The listing builds one solid part. Answer for the finished solid, in the listing's coordinates (mm). Face numbers are marked on the shaded views. A direction names the side the tool comes from. Round coordinates to 2 decimals unless told otherwise and drop trailing zeros. Write each loop counter-clockwise with the first axis right and the second up, starting at its lowest first coordinate (ties: lowest second). Pieces come first, ordered by that corner, then holes. Notation, with made-up numbers: (66.5, -8.5) - (92.5, -8.5) arc R20 ccw to (92.5, -1.5) - close; hole circle Ø1 at (5, -9). An arc over 180 degrees is marked (long way). Answer as CSV lines item,"result". Start each with the question number.
Item 1: A cutting plane is placed at D-D on z = 42. Determine the outline of the cut face in (x, y), and give its area (3 significant figures).
Item 2: Flat-ended cylindrical pins translate along their axes: pin 1 (3 mm diameter, centred on x = -52.75, y = -52.75, fed in from +Z) (3 decimals); pin 2 (2 mm diameter, centred on x = 10.5, y = 19, fed in from +Z); pin 3 (12 mm diameter, centred on x = -2, y = 4, fed in from +Z); pin 4 (5 mm diameter, centred on y = 22, z = 11.5, fed in from +X). Find the tip coordinate at first contact, or state that the pin passes through.
Item 3: A cutting plane is placed at A-A on z = 66.5. Determine the outline of the cut face in (x, y), and give its area (4 significant figures).
Item 4: A cutting plane is placed at B-B on x = 21.5. Determine the outline of the cut face in (y, z).
Item 5: A cutting plane is placed at C-C on y = 28. State how many separate pieces and enclosed holes the cut face has, and give its area (3 significant figures).
Item 6: Which of the six approach directions +Z, -Z, +X, -X, +Y, -Y give full straight-line access (tool end or side, diameter ignored) to the marked faces 1, 2 and 3?
Item 7: Straight lines are drawn through the part: line 1 along Y through (x, z) = (52.75, 1.15); line 2 along Z through (x, y) = (-13, 28.5); line 3 along X through (y, z) = (52, 1). For each, find the intervals that lie inside material, in ascending order. Write a range as [from, to].
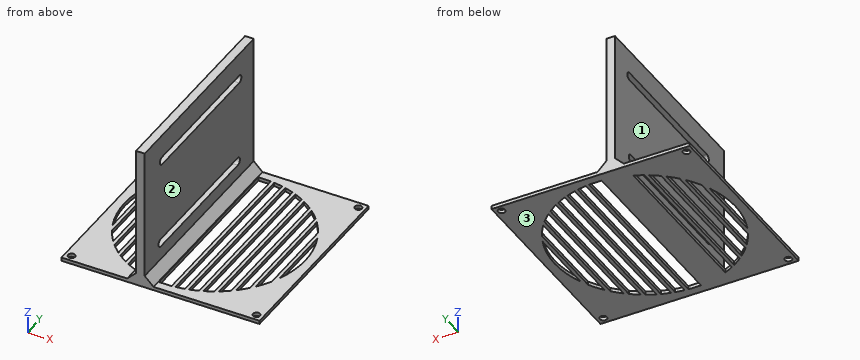
```python
from build123d import *

# Parameters (mm, degrees)
F0_W     = 113
F0_H     = 113
F0_R     = 2
F0_W_2   = 7.1751601063
F0_H_2   = 103.030346334
F1_DEPTH = 2
F2_W     = 5
F2_H     = 113
F3_DEPTH = 80
F5_DEPTH = 25
F6_SIZE  = 5


with BuildPart() as f1:
    # F0 (on Top) → F1 (new body)
    with BuildSketch(Plane.XY):
        Rectangle(F0_W, F0_H)
        with Locations((-52.75, -52.75)):
            Circle(F0_R, mode=Mode.SUBTRACT)
        with BuildLine():
            ThreePointArc((-47.5875800531, -19.6893937105), (-51.5, 0), (-47.5875800531, 19.6893937105))
            Line((-47.5875800531, 19.6893937105), (-47.5875800531, -19.6893937105))
        make_face(mode=Mode.SUBTRACT)
        with Locations((52.75, -52.75)):
            Circle(F0_R, mode=Mode.SUBTRACT)
        with BuildLine():
            Line((45.5875800531, 23.9587675998), (45.5875800531, -23.9587675998))
            ThreePointArc((45.5875800531, -23.9587675998), (43.2610879903, -27.9415150967), (40.5875800531, -31.7001316311))
            Line((40.5875800531, -31.7001316311), (40.5875800531, 31.7001316311))
            ThreePointArc((40.5875800531, 31.7001316311), (43.2610879903, 27.9415150967), (45.5875800531, 23.9587675998))
        make_face(mode=Mode.SUBTRACT)
        with BuildLine():
            Line((-45.5875800531, -23.9587675998), (-45.5875800531, 23.9587675998))
            ThreePointArc((-45.5875800531, 23.9587675998), (-43.2610879903, 27.9415150967), (-40.5875800531, 31.7001316311))
            Line((-40.5875800531, 31.7001316311), (-40.5875800531, -31.7001316311))
            ThreePointArc((-40.5875800531, -31.7001316311), (-43.2610879903, -27.9415150967), (-45.5875800531, -23.9587675998))
        make_face(mode=Mode.SUBTRACT)
        with BuildLine():
            Line((-38.5875800531, -34.106431441), (-38.5875800531, 34.106431441))
            ThreePointArc((-38.5875800531, 34.106431441), (-36.1717921774, 36.6585794962), (-33.5875800531, 39.0400367082))
            Line((-33.5875800531, 39.0400367082), (-33.5875800531, -39.0400367082))
            ThreePointArc((-33.5875800531, -39.0400367082), (-36.1717921774, -36.6585794962), (-38.5875800531, -34.106431441))
        make_face(mode=Mode.SUBTRACT)
        with BuildLine():
            Line((-31.5875800531, -40.6752355419), (-31.5875800531, 40.6752355419))
            ThreePointArc((-31.5875800531, 40.6752355419), (-29.1381205687, 42.4643371516), (-26.5875800531, 44.1061286775))
            Line((-26.5875800531, 44.1061286775), (-26.5875800531, -44.1061286775))
            ThreePointArc((-26.5875800531, -44.1061286775), (-29.1381205687, -42.4643371516), (-31.5875800531, -40.6752355419))
        make_face(mode=Mode.SUBTRACT)
        with BuildLine():
            Line((-24.5875800531, -45.2515293347), (-24.5875800531, 45.2515293347))
            ThreePointArc((-24.5875800531, 45.2515293347), (-22.1195608355, 46.5077953513), (-19.5875800531, 47.6295780756))
            Line((-19.5875800531, 47.6295780756), (-19.5875800531, -47.6295780756))
            ThreePointArc((-19.5875800531, -47.6295780756), (-22.1195608355, -46.5077953513), (-24.5875800531, -45.2515293347))
        make_face(mode=Mode.SUBTRACT)
        with Locations((-52.75, 52.75)):
            Circle(F0_R, mode=Mode.SUBTRACT)
        Rectangle(F0_W_2, F0_H_2, mode=Mode.SUBTRACT)
        with BuildLine():
            Line((5.5875800531, -51.1959856742), (5.5875800531, 51.1959856742))
            ThreePointArc((5.5875800531, 51.1959856742), (8.0973684903, 50.8594398665), (10.5875800531, 50.3999320299))
            Line((10.5875800531, 50.3999320299), (10.5875800531, -50.3999320299))
            ThreePointArc((10.5875800531, -50.3999320299), (8.0973684903, -50.8594398665), (5.5875800531, -51.1959856742))
        make_face(mode=Mode.SUBTRACT)
        with BuildLine():
            Line((17.5875800531, 48.4037914618), (17.5875800531, -48.4037914618))
            ThreePointArc((17.5875800531, -48.4037914618), (15.1070683132, -49.2344034896), (12.5875800531, -49.9379898314))
            Line((12.5875800531, -49.9379898314), (12.5875800531, 49.9379898314))
            ThreePointArc((12.5875800531, 49.9379898314), (15.1070683132, 49.2344034896), (17.5875800531, 48.4037914618))
        make_face(mode=Mode.SUBTRACT)
        with BuildLine():
            Line((24.5875800531, 45.2515293347), (24.5875800531, -45.2515293347))
            ThreePointArc((24.5875800531, -45.2515293347), (22.1195608355, -46.5077953513), (19.5875800531, -47.6295780756))
            Line((19.5875800531, -47.6295780756), (19.5875800531, 47.6295780756))
            ThreePointArc((19.5875800531, 47.6295780756), (22.1195608355, 46.5077953513), (24.5875800531, 45.2515293347))
        make_face(mode=Mode.SUBTRACT)
        with BuildLine():
            Line((26.5875800531, -44.1061286775), (26.5875800531, 44.1061286775))
            ThreePointArc((26.5875800531, 44.1061286775), (29.1381205687, 42.4643371516), (31.5875800531, 40.6752355419))
            Line((31.5875800531, 40.6752355419), (31.5875800531, -40.6752355419))
            ThreePointArc((31.5875800531, -40.6752355419), (29.1381205687, -42.4643371516), (26.5875800531, -44.1061286775))
        make_face(mode=Mode.SUBTRACT)
        with BuildLine():
            Line((33.5875800531, -39.0400367082), (33.5875800531, 39.0400367082))
            ThreePointArc((33.5875800531, 39.0400367082), (36.1717921774, 36.6585794962), (38.5875800531, 34.106431441))
            Line((38.5875800531, 34.106431441), (38.5875800531, -34.106431441))
            ThreePointArc((38.5875800531, -34.106431441), (36.1717921774, -36.6585794962), (33.5875800531, -39.0400367082))
        make_face(mode=Mode.SUBTRACT)
        with BuildLine():
            Line((47.5875800531, -19.6893937105), (47.5875800531, 19.6893937105))
            ThreePointArc((47.5875800531, 19.6893937105), (51.5, 0), (47.5875800531, -19.6893937105))
        make_face(mode=Mode.SUBTRACT)
        with Locations((52.75, 52.75)):
            Circle(F0_R, mode=Mode.SUBTRACT)
    extrude(amount=F1_DEPTH)

    # F2 (on face) → F3 (join)
    with BuildSketch(Plane.XY.offset(2)):
        with Locations((-11.5047348663, 0)):
            Rectangle(F2_W, F2_H)
    extrude(amount=F3_DEPTH)

    # F4 (on face) → F5 (cut)
    with BuildSketch(Plane.YZ.offset(-9.0047348663)):
        with BuildLine():
            Line((-35.5, 19.25), (-40, 19.25))
            ThreePointArc((-40, 19.25), (-42.25, 17), (-40, 14.75))
            Line((-40, 14.75), (-35.5, 14.75))
            Line((-35.5, 14.75), (35.5, 14.75))
            Line((35.5, 14.75), (40, 14.75))
            ThreePointArc((40, 14.75), (42.25, 17), (40, 19.25))
            Line((40, 19.25), (35.5, 19.25))
            Line((35.5, 19.25), (-35.5, 19.25))
        make_face()
        with BuildLine():
            Line((-34.5, 68.75), (-38.5, 68.75))
            ThreePointArc((-38.5, 68.75), (-40.75, 66.5), (-38.5, 64.25))
            Line((-38.5, 64.25), (-34.5, 64.25))
            Line((-34.5, 64.25), (34.5, 64.25))
            Line((34.5, 64.25), (41.5, 64.25))
            ThreePointArc((41.5, 64.25), (43.75, 66.5), (41.5, 68.75))
            Line((41.5, 68.75), (34.5, 68.75))
            Line((34.5, 68.75), (-34.5, 68.75))
        make_face()
    extrude(amount=-F5_DEPTH, mode=Mode.SUBTRACT)

    # F6
    f6_edges = [f1.edges().sort_by_distance(p)[0] for p in [
        (-9.004735, 0, 2),
        (-14.004735, 0, 2),
    ]]
    chamfer(f6_edges, length=F6_SIZE)


solid = f1.part
```
Geometry says:
1,outline,"(-14, -56.5) - (-9, -56.5) - (-9, 56.5) - (-14, 56.5) - close"
1,area,"565 mm^2"
2,pin 1,"passes through"
2,pin 2,"stops at z = 2"
2,pin 3,"stops at z = 6"
2,pin 4,"stops at x = -9"
3,outline,"(-14, -56.5) - (-9, -56.5) - (-9, -40.75) - (-14, -40.75) - close; (-14, 43.75) - (-9, 43.75) - (-9, 56.5) - (-14, 56.5) - close"
3,area,"142.5 mm^2"
4,outline,"(-56.5, 0) - (-46.8, 0) - (-46.8, 2) - (-56.5, 2) - close; (46.8, 0) - (56.5, 0) - (56.5, 2) - (46.8, 2) - close"
5,separate pieces,"14"
5,enclosed holes,"0"
5,area,"501 mm^2"
6,face 1,"+Z, -X, +Y, -Y"
6,face 2,"+Z, +X, +Y, -Y"
6,face 3,"-Z, +X, -X, +Y, -Y"
7,line 1,"y = [-56.5, -54.75], [-50.75, 50.75], [54.75, 56.5]"
7,line 2,"z = [0, 14.75], [19.25, 64.25], [68.75, 82]"
7,line 3,"x = [-56.5, -54.6], [-50.9, 50.9], [54.6, 56.5]"
